Input: dimensioned drawing with shaded views. Units: mm. Origin: part minimum x, y, z. A direction names the side the tool comes from. Give positions to 0.01 mm unless a question says otherwise; leave off trailing zeros. Order: outer loops, then holes, each group sorted by start corner. A loop starts at its lowest first (then second) coordinate and runs counter-clockwise, first axis right, second up. Notation, with made-up numbers: (47, 80) - (103, 80) arc R28 ccw to (103, 100) - close; hole circle Ø6 at (77.25, 40). An arc over 180 degrees is marked (long way). Use a Markdown table: item, result.
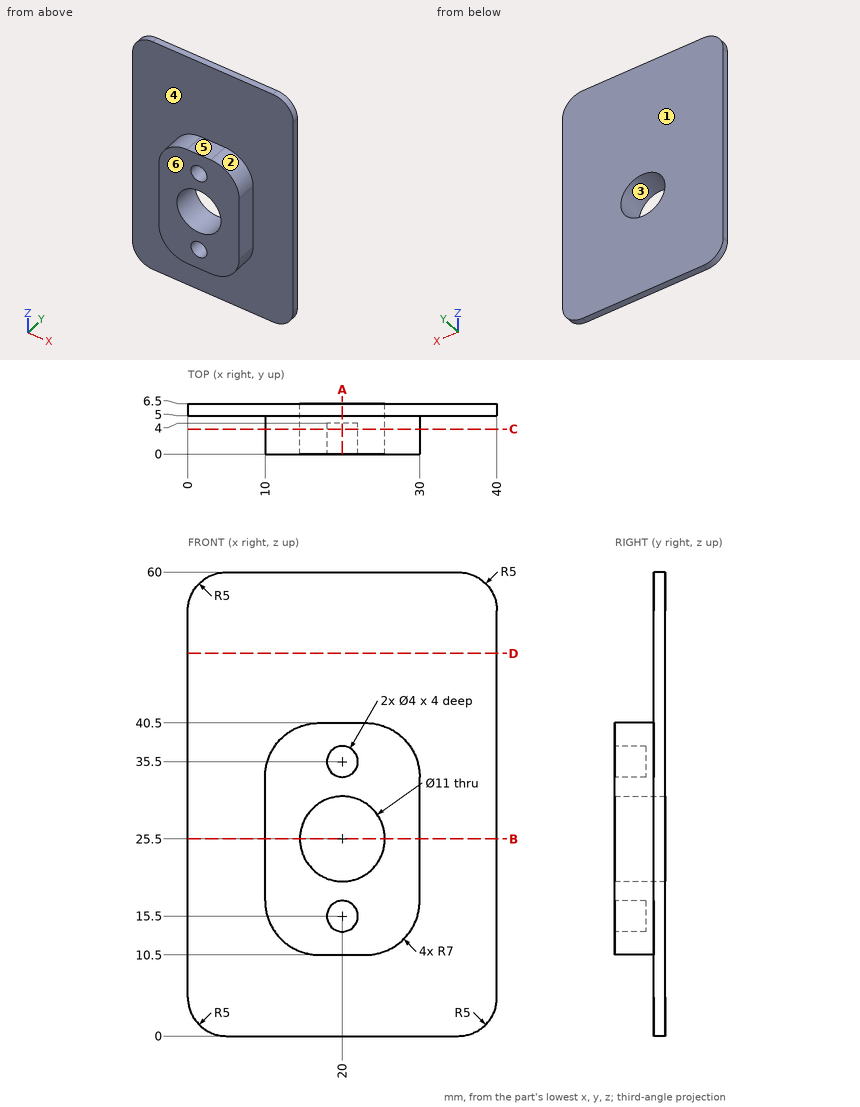
1. Pin query (flat end, axial travel): pin 1 (3 mm diameter, centred on y = 3, z = 35, fed in from -X); pin 2 (8 mm diameter, centred on x = 4.5, z = 23.5, fed in from -Y); pin 3 (1.5 mm diameter, centred on x = 19, y = 3.5, fed in from -Z). Return the tip coordinate at first contact, or that it passes through.
Response:
| item | result |
|---|---|
| pin 1 | stops at x = 10 |
| pin 2 | stops at y = 5 |
| pin 3 | stops at z = 10.5 |
2. Section query C-C (y = 3.25). Return loops of the section in (x, z).
Response:
| item | result |
|---|---|
| outline | (10, 17.5) arc R7 ccw to (17, 10.5) - (23, 10.5) arc R7 ccw to (30, 17.5) - (30, 33.5) arc R7 ccw to (23, 40.5) - (17, 40.5) arc R7 ccw to (10, 33.5) - close; hole circle Ø11 at (20, 25.5); hole circle Ø4 at (20, 15.5); hole circle Ø4 at (20, 35.5) |
3. Set-up query: the marked faces 4, 5 and 6. Return all of +Z, -Z, +X, -X, +Y, -Y with unobstructed straight access to the full face (end or side cutting, diameter ignored); none if empty.
Response:
| item | result |
|---|---|
| face 4 | -Y |
| face 5 | +Z, +X, -X, -Y |
| face 6 | +Z, -Z, +X, -X, -Y |
4. Mould query, pull axis X, two halves, no side actions, for the marked faces 1, 2 and 3. Classes: pulls with the +X half, pulls with the -X half, needs draft (parallel to the pull), parting line crosses it, or undercut.
Response:
| item | result |
|---|---|
| face 1 | needs draft |
| face 2 | pulls with the +X half |
| face 3 | undercut |
5. Material intervals for line 1 along Z through (x, y) = (20, 1.8); line 2 along X through (y, z) = (6, 28.5); line 3 along X through (y, z) = (3.5, 17), sorted ascending.
Response:
| item | result |
|---|---|
| line 1 | z = 10.5 to 13.5, 17.5 to 20, 31 to 33.5, 37.5 to 40.5 |
| line 2 | x = 0 to 15.39, 24.61 to 40 |
| line 3 | x = 10.02 to 18.68, 21.32 to 29.98 |
6. Section query D-D (z = 49.5). Return loops of the section in (x, y).
Response:
| item | result |
|---|---|
| outline | (0, 5) - (40, 5) - (40, 6.5) - (0, 6.5) - close |
7. Section query B-B (z = 25.5). Return loops of the section in (x, y), then the cut area to 3 significant figures.
Response:
| item | result |
|---|---|
| outline | (0, 5) - (10, 5) - (10, 0) - (14.5, 0) - (14.5, 6.5) - (0, 6.5) - close; (25.5, 0) - (30, 0) - (30, 5) - (40, 5) - (40, 6.5) - (25.5, 6.5) - close |
| area | 88.5 mm^2 |
8. Section query A-A (x = 20). Return loops of the section in (y, z).
Response:
| item | result |
|---|---|
| outline | (0, 10.5) - (5, 10.5) - (5, 0) - (6.5, 0) - (6.5, 20) - (0, 20) - (0, 17.5) - (4, 17.5) - (4, 13.5) - (0, 13.5) - close; (0, 31) - (6.5, 31) - (6.5, 60) - (5, 60) - (5, 40.5) - (0, 40.5) - (0, 37.5) - (4, 37.5) - (4, 33.5) - (0, 33.5) - close |
